from build123d import *

# Parameters (mm, degrees)
CROQUIS1_W              = 48
CROQUIS1_H              = 17
SALIENTE_EXTRUIR1_DEPTH = 10
CROQUIS7_W              = 9.346110156
CROQUIS7_H              = 15.524186193
CORTAR_EXTRUIR1_DEPTH   = 49


with BuildPart() as part:
    # Croquis1 → Saliente-Extruir1 (new body)
    with BuildSketch(Plane.XY):
        Rectangle(CROQUIS1_W, CROQUIS1_H)
    extrude(amount=SALIENTE_EXTRUIR1_DEPTH)

    # Croquis7 → Cortar-Extruir1 (cut, through all)
    with BuildSketch(Plane.ZY.offset(24)):
        with Locations((4.673055078, -0.737906903)):
            Rectangle(CROQUIS7_W, CROQUIS7_H)
    extrude(amount=-CORTAR_EXTRUIR1_DEPTH, mode=Mode.SUBTRACT)

    # Croquis12 → Taladro de margen para M3.53 (revolve, cut)
    with BuildSketch(Plane(origin=(15.750802653, 0, 9.346110156), x_dir=(0, 1, 0), z_dir=(1, 0, 0))):
        Polygon((0, 0), (0, 0.653889844), (1.95, 0.653889844), (1.95, 2.172799743), (4.2, 0), align=None)
    revolve(axis=Axis((15.750802653, 0, 2.996110156), (0, 0, 1)), mode=Mode.SUBTRACT)


solid = part.part
The listing builds one solid part. Answer for the finished solid, in the listing's coordinates (mm). A direction names the side the tool comes from. Give positions to 0.01 mm unless a question says otherwise; leave off trailing zeros. Write each loop counter-clockwise with the first axis right and the second up, starting at its lowest first coordinate (ties: lowest second). Pieces come first, ordered by that corner, then holes.
Item 1: Section A-A, the plane y = 0 is taken. Write down the section's boundary in (x, z), plus the area to 3 significant figures.
Item 2: Which of the six approach directions +Z, -Z, +X, -X, +Y, -Y give full straight-line access (tool end or side, diameter ignored) to faces 1 (the flat face through (0, -1, 9.346)), 2 (the flat face through (24, 3.7, 9.8))?
Item 3: Section D-D, the plane z = 2.75 is taken. Write down the section's boundary in (x, y).
Item 4: Flat-ended cylindrical pins translate along their axes: P1, Ø3, axis at x = 7.5, z = 4, coming from the -Y side; P2, Ø3, axis at x = -8.5, y = 4, coming from the -Z side. Find the tip coordinate at first contact, or state that the pin passes through.
Item 5: Section C-C, the plane y = -5.5 is taken. Write down the section's boundary in (x, z), plus the area to 3 significant figures.
Item 6: Find the intervals of material crossed by line 1 along Z through (x, y) = (3, -0.5); line 2 along Y through (x, z) = (-10.5, 1.5), in increasing order.
Item 7: Section B-B, the plane x = -16 is taken. Write down the section's boundary in (y, z).
Completed:
1. outline: (-24, 9.35) - (11.55, 9.35) - (12.23, 10) - (-24, 10) - close; (19.27, 10) - (19.95, 9.35) - (24, 9.35) - (24, 10) - close
1. area: 26.3 mm2
2. face 1: -Z, +X, -X, -Y
2. face 2: +Z, -Z, +X, +Y, -Y
3. outline: (-24, 7.02) - (24, 7.02) - (24, 8.5) - (-24, 8.5) - close
4. P1: stops at y = 7.02
4. P2: stops at z = 9.35
5. outline: (-24, 9.35) - (24, 9.35) - (24, 10) - (-24, 10) - close
5. area: 31.4 mm2
6. line 1: z = 9.35 to 10
6. line 2: y = 7.02 to 8.5
7. outline: (-8.5, 9.35) - (7.02, 9.35) - (7.02, 0) - (8.5, 0) - (8.5, 10) - (-8.5, 10) - close
